Input: part model. Units: mm. Frame: model coordinates. Coordinates: 2 decimals unless noted, no trailing zeros. Loops run counter-clockwise (first coordinate to the right, second up) from the corner with the lowest first, then second, coordinate; pieces in that order, holes last. Notation, with made-up numbers: (0.25, 46) - (9.25, 46) arc R17 ccw to (9.25, 72) - close; hole circle Ø9 at (2, 24). An arc over 180 degrees is marked (long way). Use one line per item in the form item = value.
Autodesk Inventor part; units mm, degrees
ref_plane "YZ Plane" through (0, 0, 0) normal (1, 0, 0) x (0, 1, 0)
ref_plane "XZ Plane" through (0, 0, 0) normal (0, 1, 0) x (-1, 0, 0)
ref_plane "XY Plane" through (0, 0, 0) normal (0, 0, 1) x (1, 0, 0)
sketch "Sketch1" plane through (0, 0, 0) normal (1, 0, 0) x (0, 1, 0)
  line L0 (-157.5, -42.5) -> (62.5, -42.5)
  line L1 (62.5, -42.5) -> (62.5, -262.5)
  line L2 (62.5, -262.5) -> (157.5, -262.5)
  line L3 (-157.5, -42.5) -> (-157.5, 127.5)
  line L4 (182.5, 127.5) -> (-157.5, 127.5)
  line L5 (62.5, -262.5) -> (182.5, -262.5)
  line L6 (182.5, -262.5) -> (182.5, 127.5)
  point P0 (0, 0)
  point P1 (157.5, 127.5)
  dimension "d8" = 170
  dimension "d9" = 120
extrude "Extrusion1" add sketch "Sketch1" along normal blind 5
properties part number "Side Part" material "Pine, Southern"
Q1. Pull-direction query (X, two-part tool) for faces 1 (the flat face through (0, 48, -21)), 2 (the flat face through (5, 48, -21)); classes: pulls with the +X half, pulls with the -X half, needs draft (parallel to the pull), parting line crosses it, or undercut.
Check values:
face_1 = pulls with the -X half
face_2 = pulls with the +X half
Q2. Cut plane C-C, the plane y = -115. Return loops of the section in (x, z), then the cut area to 3 significant figures.
Check values:
outline = (0, -42.5) - (5, -42.5) - (5, 127.5) - (0, 127.5) - close
area = 850 mm²
Q3. First-contact query: P1, Ø3, axis at x = 1.5, y = 40.5, coming from the -Z side. Flat tip, straight axial feed; report the tip coordinate or a pass-through.
Check values:
P1 = -42.5
Q4. Cut plane B-B, the plane z = -189.5. Return loops of the section in (x, y).
Check values:
outline = (0, 62.5) - (5, 62.5) - (5, 182.5) - (0, 182.5) - close
Q5. Ray query, line 1 along Z through (x, y) = (3.4, 51); line 2 along Y through (x, z) = (0.7, -95). Return the intervals inside material, ascending. Write a range as [from, to].
Check values:
line_1 = [-42.5, 127.5]
line_2 = [62.5, 182.5]
Q6. Cut plane A-A, the plane x = 3.55. Return loops of the section in (y, z).
Check values:
outline = (-157.5, -42.5) - (62.5, -42.5) - (62.5, -262.5) - (182.5, -262.5) - (182.5, 127.5) - (-157.5, 127.5) - close
